Design review of the part built by this model. Coordinates are the model's own, in mm. Face numbers are marked on the shaded views. A direction names the side the tool comes from. Coordinates: 2 decimals unless noted, no trailing zeros. Write each loop counter-clockwise with the first axis right and the second up, starting at its lowest first coordinate (ties: lowest second). Pieces come first, ordered by that corner, then holes. Notation, with made-up numbers: (-25, 0) - (28, 0) arc R28 ccw to (28, 34) - close; hole circle Ø1 at (35.25, 3.25). An arc over 180 degrees is marked (long way). Answer as a JSON object with one key per item and string values.
```python
from build123d import *

# Parameters (mm, degrees)
PAD_DEPTH = 3
FILLET_R  = 0.8


with BuildPart() as part:
    # Sketch → Pad (new body)
    with BuildSketch(Plane.XY):
        with BuildLine():
            Line((-4, 12), (4, 12))
            Line((4, 12), (4, -12))
            Line((4, -12), (-4, -12))
            Line((-4, -0.75), (-4, -12))
            Line((-8, -0.75), (-4, -0.75))
            Line((-8, -16), (-8, -0.75))
            Line((-8, -16), (20, -16))
            ThreePointArc((20, -16), (25.108875, 0), (20, 16))
            Line((20, 16), (-8, 16))
            Line((-8, 16), (-8, 0.75))
            Line((-8, 0.75), (-4, 0.75))
            Line((-4, 0.75), (-4, 12))
        make_face()
        with BuildLine():
            Line((8, 12), (8, -12))
            Line((8, -12), (18, -12))
            ThreePointArc((18, -12), (21.253947, 0), (18, 12))
            Line((8, 12), (18, 12))
        make_face(mode=Mode.SUBTRACT)
    extrude(amount=PAD_DEPTH)

    # Fillet
    fillet_edges = [part.edges().sort_by_distance(p)[0] for p in [
        (21.253947, 0, 3),
        (25.108875, 0, 3),
        (25.108875, 0, 0),
        (21.253947, 0, 0),
    ]]
    fillet(fillet_edges, radius=FILLET_R)


solid = part.part
```
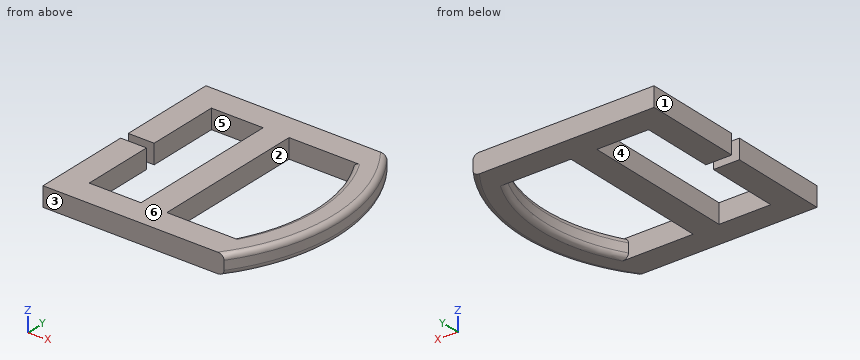
(1) Take a section at B-B, the plane z = 1.4. Write out the cut boundary in (x, y), and give its area (3 significant figures).
Solved:
{"outline": "(-8, -16) - (20, -16) arc R27.61 ccw to (20, 16) - (-8, 16) - (-8, 0.75) - (-4, 0.75) - (-4, 12) - (4, 12) - (4, -12) - (-4, -12) - (-4, -0.75) - (-8, -0.75) - close; hole (8, -12) - (18, -12) arc R23.75 ccw to (18, 12) - (8, 12) - close", "area": "516 mm^2"}
(2) Take a section at A-A, the plane x = -5. Write out the cut boundary in (y, z), and give its area (3 significant figures).
Solved:
{"outline": "(-16, 0) - (-0.75, 0) - (-0.75, 3) - (-16, 3) - close; (0.75, 0) - (16, 0) - (16, 3) - (0.75, 3) - close", "area": "91.5 mm^2"}
(3) Take a section at C-C, the plane y = -10. Give the number of separate pieces and of enclosed holes in the cut face, and give its area (3 significant figures).
Solved:
{"separate pieces": "3", "enclosed holes": "0", "area": "36.0 mm^2"}
(4) For pin 1 (1.5 mm diameter, centred on y = 8.5, z = 2, fed in from +X); pin 2 (3 mm diameter, centred on x = 18, y = 10.5, fed in from -Z); pin 3 (1.5 mm diameter, centred on y = -6, z = 2, fed in from +X), all flat-tipped, find the tip position at first contact; note any pin that passes through.
Solved:
{"pin 1": "stops at x = 24", "pin 2": "stops at z = 0", "pin 3": "stops at x = 24.61"}
(5) To check wall thickness, follow line 1 (Y direction, x = 13.5, z = 0.45); line 2 (X direction, y = 3.5, z = 2.6); line 3 (X direction, y = 2, z = 2.05). State the ranges of each line that lie inside material, in increasing order. Write a range as from..to.
Solved:
{"line 1": "y = -16..-12, 12..16", "line 2": "x = -8..-4, 4..8, 21.1..24.78", "line 3": "x = -8..-4, 4..8, 21.17..25.04"}
(6) Take a section at D-D, the plane x = 8.5. Write out the cut boundary in (y, z).
Solved:
{"outline": "(-16, 0) - (-12, 0) - (-12, 3) - (-16, 3) - close; (12, 0) - (16, 0) - (16, 3) - (12, 3) - close"}
(7) Tool access review of the marked faces 5 and 6: name each direction out of +Z, -Z, +X, -X, +Y, -Y from which nothing blocks a thin tool from reaching the whole face with its end or side.
Solved:
{"face 5": "+Z, -Z", "face 6": "+Z, +X, -X, +Y, -Y"}
(8) The part is to be moulded in two halves that separate along X. For the marked faces 1, 2, 3 and 4, say which applies: pulls with the +X half, pulls with the -X half, needs draft (parallel to the pull), parting line crosses it, or undercut.
Solved:
{"face 1": "pulls with the -X half", "face 2": "undercut", "face 3": "needs draft", "face 4": "undercut"}
